Could you check a few things on this model? Use its own coordinates, in mm. A direction names the side the tool comes from. Round coordinates to 2 decimals unless told otherwise and drop trailing zeros. Loops run counter-clockwise (first coordinate to the right, second up) from the corner with the lowest first, then second, coordinate; pieces in that order, holes last. Notation, with made-up numbers: (-26, 42) -> (5, 42) arc R33 cw to (5, 78) -> close; hole circle Ø3 at (40, -27). An arc over 180 degrees is marked (long way). Write each question's results on one line, items separated by ' | '.
from build123d import *

# Parameters (mm, degrees)
BOSS_EXTRUDE2_DEPTH            = 19.05
FILLET1_R                      = 22.225
FILLET2_R                      = 31.75
SKETCH6_W                      = 19.05
SKETCH6_H                      = 157.3
BOSS_EXTRUDE3_DEPTH            = 12.7
FILLET1_OF_MIRROR1_R           = 22.225
FILLET2_OF_MIRROR1_R           = 31.75
F_5_16_0_3125_DIAMETER_HOLE1_D = 7.9375
F_8_CLEARANCE_HOLE1_D          = 4.9149
HOLE1_D                        = 3.175
HOLE1_DEPTH                    = 31.75
HOLE1_CSINK_D                  = 10.16
HOLE1_CSINK_ANGLE              = 82
HOLE1_TIP                      = 0.953866233
HOLE2_D                        = 3.175
HOLE2_DEPTH                    = 31.75
HOLE2_CSINK_D                  = 10.16
HOLE2_CSINK_ANGLE              = 82
HOLE2_TIP                      = 0.953866233
F_1_4_0_25_DIAMETER_HOLE1_D    = 6.35


with BuildPart() as part:
    # Sketch1 → Boss-Extrude2 (new body)
    with BuildSketch(Plane.XY):
        Polygon((-341.304465963, -157.3), (-341.304465963, -175), (-186.304465963, -175), (-186.304465963, -46), (-124.004465969, -46), (-124.004465969, 12.7), (-244.004465963, 12.7), (-244.004465963, -144.6), (-341.304465963, -144.6), align=None)
    boss_extrude2 = extrude(amount=BOSS_EXTRUDE2_DEPTH)

    # Fillet1
    fillet1_edges = [part.edges().sort_by_distance(p)[0] for p in [
        (-186.304465963, -175, 9.525),
    ]]
    fillet(fillet1_edges, radius=FILLET1_R)

    # Fillet2
    fillet2_edges = [part.edges().sort_by_distance(p)[0] for p in [
        (-186.304465963, -46, 9.525),
    ]]
    fillet(fillet2_edges, radius=FILLET2_R)

    # Sketch6 → Boss-Extrude3 (add)
    with BuildSketch(Plane.ZY.offset(244.004465963)):
        with Locations((9.525, -65.95)):
            Rectangle(SKETCH6_W, SKETCH6_H)
    boss_extrude3 = extrude(amount=BOSS_EXTRUDE3_DEPTH)

    # Mirror1: Boss-Extrude2, Boss-Extrude3 across plane
    add(boss_extrude2.mirror(Plane(origin=(-124.004465969, 12.7, 19.05), x_dir=(0, 0, 1), z_dir=(1, 0, 0))))
    add(boss_extrude3.mirror(Plane(origin=(-124.004465969, 12.7, 19.05), x_dir=(0, 0, 1), z_dir=(1, 0, 0))))

    # Fillet1 of Mirror1
    fillet1_of_mirror1_edges = [part.edges().sort_by_distance(p)[0] for p in [
        (-61.704465975, -175, 9.525),
    ]]
    fillet(fillet1_of_mirror1_edges, radius=FILLET1_OF_MIRROR1_R)

    # Fillet2 of Mirror1
    fillet2_of_mirror1_edges = [part.edges().sort_by_distance(p)[0] for p in [
        (-61.704465975, -46, 9.525),
    ]]
    fillet(fillet2_of_mirror1_edges, radius=FILLET2_OF_MIRROR1_R)

    # 5/16 (0.3125) Diameter Hole1 (through all)
    with Locations(Plane(origin=(0, 0, 0), x_dir=(-1, 0, 0), z_dir=(0, 0, -1))):
        with Locations((124.004465969, -34.7475), (124.004465969, -14.4275)):
            Hole(F_5_16_0_3125_DIAMETER_HOLE1_D / 2)

    # #8 Clearance Hole1 (through all)
    with Locations(Plane.XY.offset(19.05)):
        with Locations((-111.927249911, -24.5875), (-136.081682027, -24.5875)):
            Hole(F_8_CLEARANCE_HOLE1_D / 2)

    # Hole1
    with Locations(Plane(origin=(-124.004465969, -155.024290059, 19.05), x_dir=(1, 0, 0), z_dir=(0, 0, 1))):
        with Locations((-162.299999994, -8.625709941), (-113.649999994, 50.157623392), (-113.649999994, 102.590956725), (162.299999994, -8.625709941), (113.649999994, 50.157623392), (113.649999994, 102.590956725), (63.85, 161.374290059), (0, 161.374290059), (-63.85, 161.374290059)):
            CounterSinkHole(HOLE1_D / 2, HOLE1_CSINK_D / 2, depth=HOLE1_DEPTH, counter_sink_angle=HOLE1_CSINK_ANGLE)
            with Locations((0, 0, -(HOLE1_DEPTH + HOLE1_TIP / 2))):  # 118° drill point
                Cone(0, HOLE1_D / 2, HOLE1_TIP, mode=Mode.SUBTRACT)

    # Hole2
    with Locations(Plane(origin=(-124.004465969, -155.024290059, 0), x_dir=(-1, 0, 0), z_dir=(0, 0, -1))):
        with Locations((126.349999994, 161.374290059), (146.083333327, 4.074290059), (172.166666661, 4.074290059), (126.349999994, 34.524290059), (126.349999994, 130.924290059), (-172.166666661, 4.074290059), (-146.083333327, 4.074290059), (-126.349999994, 34.524290059), (-126.349999994, 130.924290059), (-126.349999994, 161.374290059)):
            CounterSinkHole(HOLE2_D / 2, HOLE2_CSINK_D / 2, depth=HOLE2_DEPTH, counter_sink_angle=HOLE2_CSINK_ANGLE)
            with Locations((0, 0, -(HOLE2_DEPTH + HOLE2_TIP / 2))):  # 118° drill point
                Cone(0, HOLE2_D / 2, HOLE2_TIP, mode=Mode.SUBTRACT)

    # 1/4 (0.25) Diameter Hole1 (through all)
    with Locations(Plane.XY.offset(19.05)):
        with Locations((-217.016965963, -157.3), (-217.016965963, -12.7), (-30.991965975, -12.7), (-30.991965975, -157.3)):
            Hole(F_1_4_0_25_DIAMETER_HOLE1_D / 2)


solid = part.part
1) I need wall thicknesses on line 1 (X direction, y = 6.35, z = 9.75); line 2 (X direction, y = -150.95, z = 10.5); line 3 (X direction, y = -126.5, z = 11.25). Which ranges of each line are inside material? Lowest first, please.
Model answer:
line 1: x = -256.7 to -251.94, -248.77 to -189.44, -186.27 to -125.59, -122.42 to -61.74, -58.57 to 0.76, 3.93 to 8.7 | line 2: x = -341.3 to -297.76, -294.58 to -271.68, -268.5 to -186.3, -61.7 to 20.49, 23.67 to 46.57, 49.75 to 93.3 | line 3: x = -256.7 to -186.3, -61.7 to 8.7
2) I want a section at D-D, the plane x = -69.5. Write out the boundary of the cut face in (y, z).
Model answer:
outline: (-56.91, 0) -> (12.7, 0) -> (12.7, 19.05) -> (-56.91, 19.05) -> close
3) For faces 5 (the conical face through (23.023, -149.468, 3.823)), 6 (the flat face through (-256.704, -65, 9)), 7 (the flat face through (-61.704, -116, 9)), which set-ups out of +Z, -Z, +X, -X, +Y, -Y let a thin tool reach every point of the face, with its end or its side?
Model answer:
face 5: -Z | face 6: +Z, -Z, -X, +Y | face 7: +Z, -Z, -Y
4) I want a section at C-C, the plane z = 9.5. Give the number of separate pieces and of enclosed holes in the cut face, plus the area to 3 significant figures.
Model answer:
separate pieces: 1 | enclosed holes: 27 | area: 38,700 mm2
5) I want a section at A-A, the plane y = -85. Write out the boundary of the cut face in (x, z), plus the area to 3 significant figures.
Model answer:
outline: (-256.7, 0) -> (-186.3, 0) -> (-186.3, 19.05) -> (-256.7, 19.05) -> close; (-61.7, 0) -> (8.7, 0) -> (8.7, 19.05) -> (-61.7, 19.05) -> close | area: 2,680 mm2
6) I'm going to push flat-ended pins straight in: pin 1 (3 mm diameter, centred on x = -280.5, z = 2.5, fed in from +Y); pin 2 (9.5 mm diameter, centred on y = -102.5, z = 13, fed in from +X); pin 3 (9.5 mm diameter, centred on x = -129.5, z = 13.5, fed in from -Y). Where does each tip first touch, or does it pass through?
Model answer:
pin 1: stops at y = -144.6 | pin 2: stops at x = 8.7 | pin 3: stops at y = -46
7) I want a section at B-B, the plane y = -3. Write out the boundary of the cut face in (x, z), plus the area to 3 significant figures.
Model answer:
outline: (-256.7, 0) -> (8.7, 0) -> (8.7, 19.05) -> (-256.7, 19.05) -> close | area: 5,060 mm2
8) If we mould it in two halves opening along Y, with no side actions, what happens to faces 1 (the conical face through (0.59, 6.43, 3.82)), 2 (the flat face through (93.296, -160, 9)), 3 (the cylindrical face through (-55.021, -168.662, 9.658)), 4 (the flat face through (50, -144.6, 9))? For each: released by +Y, released by -Y, zero draft, split by the parting line, or undercut.
Model answer:
face 1: undercut | face 2: zero draft | face 3: released by -Y | face 4: released by +Y
